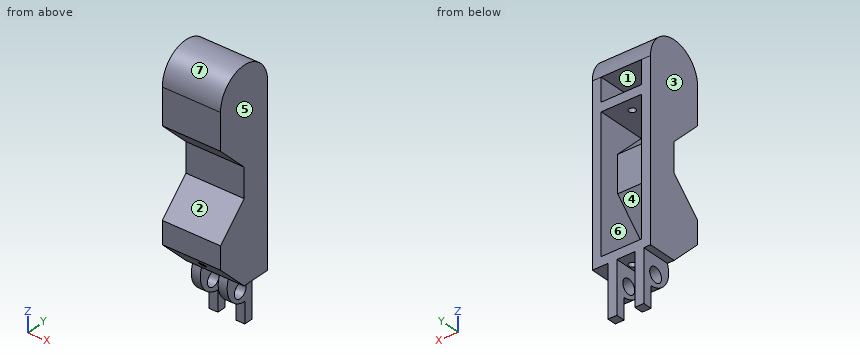
Autodesk Inventor part; units mm, degrees
ref_plane "Work Plane1" through (4.5, 0, 0) normal (1, 0, 0) x (0, 0, -1)
ref_plane "YZ Plane" through (0, 0, 0) normal (1, 0, 0) x (0, 1, 0)
ref_plane "XZ Plane" through (0, 0, 0) normal (0, 1, 0) x (-1, 0, 0)
sketch "Sketch2" plane through (0, 0, 0) normal (1, 0, 0) x (0, 1, 0)
  line L0 (0, 0) -> (0, -8)
  line L1 (13, 0) -> (13, -21)
  arc A0 (13, 0) -> (0, 0) centre (6.5, 0) ccw
  line L2 (-3.1385, 0) -> (18.8309, 0)
  line L3 (0, -58.4723) -> (0, 17.3287)
  line L4 (0, -8) -> (6.5, -14.5)
  line L5 (0, -8) -> (9.1924, -8) construction
  line L6 (6.5, -14.5) -> (6.5, -21)
  line L7 (6.5, -21) -> (0, -27.5)
  line L8 (6.5, -21) -> (15.6924, -21) construction
  line L9 (0, -27.5) -> (0, -32.5)
  line L10 (0, -32.5) -> (6.5, -39)
  line L11 (0, -32.5) -> (9.1924, -32.5) construction
  line L12 (13, -21) -> (13, -39)
  line L13 (13, -39) -> (13, -45.5)
  arc A1 (6.5, -39) -> (13, -45.5) centre (11.1419, -40.8581) ccw
  circle A2 centre (9.75, -43) radius 1.625
  dimension "d49" = 4
  dimension "d4" = 13
  dimension "d9" = 45
  dimension "d10" = 6.5
  dimension "d11" = 8
  dimension "d12" = 6.5
  dimension "d13" = 135
  dimension "d14" = 6.5
  dimension "d15" = 5
  dimension "d16" = 45
  dimension "d17" = 6.5
  dimension "d18" = 18
  dimension "d19" = 6.5
  dimension "d20" = 5
  dimension "d21" = 3.25
  dimension "d22" = 3.25
  dimension "d23" = 2.5
  dimension "d94" = 21
extrude "Extrusion1" add sketch "Sketch2" along normal mid plane 13 contours L2 L1 L12 L13 A1 L10 L3 L7 L6 L4 L0 | A0 L2
sketch "Sketch3" plane through (-6.5, 13, 0) normal (0, 1, 0) x (1, 0, 0)
  line L0 (0, 39) -> (13, 39)
  line L1 (0, 46) -> (1.5, 46)
  line L2 (1.5, 46) -> (1.5, 39)
  line L3 (1.5, 39) -> (0, 39)
  line L4 (0, 39) -> (0, 46)
  line L5 (0, 0) -> (0, 45.5)
  line L6 (3.5, 46) -> (7.5, 46)
  line L7 (7.5, 46) -> (7.5, 39)
  line L8 (7.5, 39) -> (3.5, 39)
  line L9 (3.5, 39) -> (3.5, 46)
  line L10 (9.5, 46) -> (13, 46)
  line L11 (13, 46) -> (13, 39)
  line L12 (13, 39) -> (9.5, 39)
  line L13 (9.5, 39) -> (9.5, 46)
  line L14 (13, 45.5) -> (13, 0)
  point P0 (6.5, 0)
  dimension "d47" = 1.5
  dimension "d48" = 7
  dimension "d49" = 4
  dimension "d50" = 7
  dimension "d51" = 2
  dimension "d52" = 7
  dimension "d53" = 2
extrude "Extrusion2" cut sketch "Sketch3" against normal blind 13
ref_plane "Work Plane1" through (4.5, 0, 0) normal (1, 0, 0) x (0, 0, -1)
sketch "Sketch4" plane through (4.5, 0, 0) normal (1, 0, 0) x (0, 0, -1)
  arc A0 (0, 13) -> (0, 0) centre (0, 6.5) ccw
  line L0 (0, 13) -> (39, 13)
  line L1 (39, 13) -> (39, 6.5)
  line L2 (39, 6.5) -> (32.5, 0)
  line L3 (32.5, 0) -> (27.5, 0)
  line L4 (27.5, 0) -> (21, 6.5)
  line L5 (39, 13) -> (39, 6.5)
  line L6 (39, 6.5) -> (32.5, 0)
  line L7 (32.5, 0) -> (27.5, 0)
  line L8 (27.5, 0) -> (21, 6.5)
  line L9 (21, 6.5) -> (14.5, 6.5)
  line L10 (14.5, 6.5) -> (8, 0)
  line L11 (8, 0) -> (0, 0)
  arc A1 (0, 13) -> (0, 0) centre (0, 6.5) ccw
  line L12 (0, 13) -> (39, 13)
  line L13 (0, 13) -> (0, 2)
  line L14 (0, 2) -> (5.1716, 2)
  line L15 (7.1716, 2) -> (13.6716, 8.5)
  line L16 (7.1716, 2) -> (16.364, 2) construction
  line L17 (37, 13) -> (37, 7.3284)
  line L18 (37, 7.3284) -> (31.6716, 2)
  line L19 (37, 7.3284) -> (44.5355, 7.3284) construction
  line L20 (31.6716, 2) -> (28.3284, 2)
  line L21 (28.3284, 2) -> (21.8284, 8.5)
  line L22 (28.3284, 2) -> (37.5208, 2) construction
  line L23 (21.8284, 8.5) -> (13.6716, 8.5)
  line L24 (7.1716, 2) -> (7.1716, 13)
  line L25 (5.1716, 2) -> (5.1716, 13)
  line L26 (0, 13) -> (5.1716, 13)
  line L27 (7.1716, 13) -> (37, 13)
  dimension "d57" = 11
  dimension "d58" = 2
  dimension "d59" = 45
  dimension "d60" = 2
  dimension "d62" = 2
  dimension "d63" = 2
  dimension "d64" = 135
  dimension "d65" = 2
  dimension "d66" = 2
  dimension "d67" = 135
  dimension "d95" = 2
  dimension "d96" = 2
extrude "Extrusion3" cut sketch "Sketch4" against normal blind 9 contours L0 L25 L14 L13 | L0 L17 L18 L20 L21 L23 L15 L24
sketch "Sketch5" plane through (4.5, 2, -7.1716) normal (0, 0, -1) x (-1, 0, 0)
  line L0 (0, 11) -> (0, 1)
  line L1 (9, 1) -> (9, 11)
  line L2 (0, 11) -> (0, 0)
  line L3 (9, 0) -> (9, 11)
  line L4 (0, 11) -> (9, 11)
  circle A0 centre (4.5, 8) radius 0.75
  circle A1 centre (4.5, 3) radius 0.75
  line L5 (0, 0) -> (9, 0)
  point P0 (4.5, -2)
  dimension "d72" = 1.5
  dimension "d73" = 4.5
  dimension "d74" = 3
  dimension "d75" = 1.5
  dimension "d77" = 4.5
extrude "Extrusion4" cut sketch "Sketch5" against normal blind 2 contours A0 | A1
sketch "Sketch6" plane through (1, 13, -39) normal (0, 0, -1) x (-1, 0, 0)
  line L0 (1, -15.6) -> (1, 2.6)
  line L1 (10.1, -13) -> (-8.1, -13)
  circle A0 centre (1, -3) radius 0.75
  line L2 (0, 0) -> (4, 0)
  circle A1 centre (1, -10) radius 0.75
  point P0 (1, -13)
  dimension "d80" = 1.5
  dimension "d81" = 3
  dimension "d82" = 1.5
  dimension "d83" = 3
extrude "Extrusion5" cut sketch "Sketch6" against normal blind 9
sketch "Sketch7" plane through (3, 13, -39) normal (1, 0, 0) x (0, 0, -1)
  line L0 (6.5, 0) -> (0, 0)
  line L1 (6.5, 0) -> (11.5, 0)
  line L2 (11.5, 0) -> (11.5, -2)
  line L3 (11.5, -2) -> (6.5, -2)
  line L4 (6.5, -2) -> (6.5, 0)
  point P0 (-39, -13)
  dimension "d86" = 5
  dimension "d87" = 2
extrude "Extrusion6" add sketch "Sketch7" against normal blind 2
sketch "Sketch8" plane through (-5, 13, -45.5) normal (-1, 0, 0) x (0, 0, 1)
  line L0 (0, 0) -> (6.5, 0)
  line L1 (-5, -2) -> (0, -2)
  line L2 (0, -2) -> (0, 0)
  line L3 (0, 0) -> (-5, 0)
  line L4 (-5, 0) -> (-5, -2)
  point P0 (45.5, -13)
  dimension "d90" = 5
  dimension "d91" = 2
extrude "Extrusion7" add sketch "Sketch8" against normal blind 2
properties part number "middle"
Input: part model. Units: mm. Frame: model coordinates. Face numbers are marked on the shaded views. A direction names the side the tool comes from. Give positions to 0.01 mm unless a question says otherwise; leave off trailing zeros. Order: outer loops, then holes, each group sorted by start corner. A loop starts at its lowest first (then second) coordinate and runs counter-clockwise, first axis right, second up. Notation, with made-up numbers: (41, -21.5) - (67, -21.5) arc R19 cw to (67, 6.5) - close; hole circle Ø5 at (30.5, -13.75). An arc over 180 degrees is marked (long way). Put each result on its own line as item: value.
Item 1: Ray query, L1, parallel to Z at x = -4.25, y = 8; L2, parallel to Z at x = -2, y = 9.25; L3, parallel to X at y = 3, z = -34.6. Return the intervals inside material, ascending. Write a range as from..to.
Found:
L1: z = -44.75..-37, -22.33..-13.17, -7.17..-5.17, 0..6.32
L2: z = -39..-37, -7.17..-5.17, 0..5.89
L3: x = -6.5..-0.75, 0.75..6.5
Item 2: Section query D-D, the plane y = 10. Count the separate pieces of the cut face and the enclosed holes in it, then the cut area to 3 significant figures.
Found:
separate pieces: 3
enclosed holes: 0
area: 271 mm^2
Item 3: Access query for the marked faces 1, 2 and 3. Directions: +Z, -Z, +X, -X, +Y, -Y. A direction counts if a zero-diameter tool reaches every point of the face in a straight line with its end or side. Return the directions, or none.
Found:
face 1: +Y
face 2: +X, -X, -Y
face 3: +Z, -Z, -X, +Y, -Y
Item 4: Section query A-A, the plane y = 3. Return loops of the section in (x, z).
Found:
outline: (-6.5, -35.5) - (-0.75, -35.5) - (-0.75, -32.67) - (-4.5, -32.67) - (-4.5, -27.33) - (4.5, -27.33) - (4.5, -32.67) - (0.75, -32.67) - (0.75, -35.5) - (6.5, -35.5) - (6.5, -24.5) - (-6.5, -24.5) - close; (-6.5, -11) - (6.5, -11) - (6.5, 5.48) - (-6.5, 5.48) - close; hole (-4.5, -8.17) - (4.5, -8.17) - (4.5, -7.17) - (-4.5, -7.17) - close; hole (-4.5, -5.17) - (4.5, -5.17) - (4.5, 0) - (-4.5, 0) - close
Item 5: Section query C-C, the plane z = -40. Return loops of the section in (x, y), then the cut area to 3 significant figures.
Found:
outline: (-5, 6.22) - (-3, 6.22) - (-3, 13) - (-5, 13) - close; (1, 6.22) - (3, 6.22) - (3, 13) - (1, 13) - close
area: 27.1 mm^2
Item 6: Section query B-B, the plane z = -29. Return loops of the section in (x, y), then the cut area to 3 significant figures.
Found:
outline: (-6.5, 0) - (6.5, 0) - (6.5, 13) - (4.5, 13) - (4.5, 2) - (-4.5, 2) - (-4.5, 13) - (-6.5, 13) - close
area: 70.0 mm^2
Item 7: Draft query along Z for the marked faces 4, 5, 6 and 7. Return one class per face: +Z half, -Z half, draft (parallel to the pull), parting line (faces both ways), or undercut.
Found:
face 4: undercut
face 5: draft
face 6: undercut
face 7: +Z half
Item 8: Contact query for flat-ended pins moving along their axis: pin 1 (3 mm diameter, centred on x = 0, y = 9, fed in from +Z); pin 2 (4 mm diameter, centred on x = 2, z = -10.5, fed in from +Y); pin 3 (1.2 mm diameter, centred on x = -5.5, y = 10.5, fed in from -Z). Output: stop coordinate, or through.
Found:
pin 1: stops at z = 6.42
pin 2: stops at y = 7.33
pin 3: stops at z = -45.85
